Source: CAD feature listing. Evaluate the final solid. Frame: model axes, mm. A direction names the side the tool comes from. Coordinates: 2 decimals unless noted, no trailing zeros. Order: outer loops, then holes, each group sorted by start corner. A loop starts at its lowest first (then second) coordinate and runs counter-clockwise, first axis right, second up.
Item 1: Reachability of faces 4 (the flat face through (-66, 2, 0)), 5 (the cylindrical face through (-90.785, 1.565, -88.81)) from +Z, -Z, +X, -X, +Y, -Y: full face, straight path, thin tool, end or side. Return the list, or none.
Item 2: Mould query, pull axis Z, two halves, no side actions, for faces 1 (the cylindrical face through (4.34, 1.61, 4.636)), 2 (the flat face through (0, 2, -66)), 3 (the cylindrical face through (1.93, 1.61, 2.52)). Classes: released by +Z, released by -Z, zero draft, split by the parting line, or undercut.
Item 3: Contact query for flat-ended pins moving along their axis: P1, Ø1.6, axis at y = 2, z = -74, coming from the +X side; P2, Ø1, axis at x = -17, y = 2.5, coming from the -Z side. Output: stop coordinate, or through.
Item 4: Section B-B on x = -78. Return the cut outline in (y, z) (3 decimals).
Item 5: Section C-C on z = -95. Return the cut outline in (x, y) (3 decimals), then the cut area to 3 significant figures.
Item 6: Ray query, line 1 (X direction, y = 0.9, z = -0.5); line 2 (X direction, y = 2.75, z = -2); line 3 (X direction, y = 0.4, z = -110.5). Return the intervals inside material, ascending.
Item 7: Section A-A on y = 1.85. Return the cut outline in (x, z) (3 decimals).
Autodesk Inventor part; units mm, degrees
ref_plane "YZ Plane" through (0, 0, 0) normal (1, 0, 0) x (0, 1, 0)
ref_plane "XZ Plane" through (0, 0, 0) normal (0, 1, 0) x (-1, 0, 0)
ref_plane "XY Plane" through (0, 0, 0) normal (0, 0, 1) x (1, 0, 0)
sketch "Sketch5" plane through (0, 0, 0) normal (0, 1, 0) x (-1, 0, 0)
  line L0 (0, 0) -> (127, 0) construction
  circle A0 centre (0, 0) radius 127
  line L1 (0, 0) -> (127, 0)
  line L2 (0, 0) -> (0, -127)
  dimension "d27" = 254
extrude "Extrusion2" add sketch "Sketch5" along normal blind 3.175
sketch "Sketch6" plane through (0, 3.175, 0) normal (0, 1, 0) x (1, 0, 0)
  circle A0 centre (0, 0) radius 127
  line L0 (0, 0) -> (-127, 0)
  line L1 (0, 0) -> (0, 127)
  line L2 (-127, 0) -> (-147.1811, -31.5463)
  line L3 (-147.1811, -31.5463) -> (-90.1509, -154.4564)
  line L4 (-90.1509, -154.4564) -> (47.5084, -160.3561)
  line L5 (47.5084, -160.3561) -> (160.365, -93.0014)
  line L6 (160.365, -93.0014) -> (183.4453, 199.208)
  line L7 (183.4453, 199.208) -> (0, 127)
extrude "Extrusion3" cut sketch "Sketch6" against normal blind 3.175 contours A0 L0 L1 picked at (43.7214, -72.324)
sketch "Sketch9" plane through (0, 3.175, 0) normal (0, 1, 0) x (1, 0, 0)
  circle A0 centre (0, 0) radius 6.35
  circle A1 centre (0, 0) radius 3.175
  dimension "d37" = 12.7
  dimension "d38" = 6.35
extrude "Extrusion5" add sketch "Sketch9" against normal blind 3.175
sketch "Sketch10" plane through (0, 3.175, 0) normal (0, 1, 0) x (1, 0, 0)
  circle A0 centre (0, 0) radius 3.175
  dimension "d41" = 6.35
extrude "Extrusion6" cut sketch "Sketch10" against normal blind 6.35
sketch "Sketch11" plane through (0, 3.175, 0) normal (0, 1, 0) x (1, 0, 0)
  arc A0 (0, 127) -> (-127, 0) centre (0, 0) ccw
  arc A1 (0, 127) -> (0, 127) centre (0, 0) ccw
  line L0 (-127, 0) -> (0, 0)
  line L1 (-127, 0) -> (0, 0)
  line L2 (-120.7842, 39.2452) -> (0, 0)
  circle A2 centre (0, 0) radius 3.175
  line L3 (-102.7452, 74.6487) -> (0, 0)
  line L4 (0, 0) -> (-74.6487, 102.7452)
  line L5 (-39.2452, 120.7842) -> (0, 0)
  point P0 (0, 127)
  dimension "d52" = 90
equation "\"d42\" = d41"
properties part number "swiweller"
Answer list:
1. face 4: +Z, -X, +Y, -Y
1. face 5: -Z, -X, +Y, -Y
2. face 1: split by the parting line
2. face 2: zero draft
2. face 3: undercut
3. P1: stops at x = 0
3. P2: stops at z = -125.92
4. outline: (0, -100.225) - (3.175, -100.225) - (3.175, 0) - (0, 0) - close
5. outline: (-84.285, 0) - (0, 0) - (0, 3.175) - (-84.285, 3.175) - close
5. area: 268 mm2
6. line 1: x = -127 to -3.14, 3.14 to 6.33
6. line 2: x = -126.98 to -2.47, 2.47 to 6.03
6. line 3: x = -62.6 to 0
7. outline: (-127, 0) arc R127 ccw to (0, -127) - (0, -6.35) arc R6.35 ccw (long way) to (-6.35, 0) - close; hole circle Ø6.35 at (0, 0)
